Geometry check sheet. Reference: drawing and pictorial views, mm from the part's lowest x, y, z. A direction names the side the tool comes from. Coordinates: 2 decimals unless noted, no trailing zeros. Write each loop counter-clockwise with the first axis right and the second up, starting at its lowest first coordinate (ties: lowest second). Pieces come first, ordered by that corner, then holes. Notation, with made-up numbers: (58, 78) - (114, 78) arc R23 cw to (114, 99) - close; hole circle Ø2 at (4.5, 42). An arc over 180 degrees is marked (long way). Use one line per item in the form item = value. Start each with the question number.
(1) Sectioned sample at A-A (x = 7.5). Record the cut outline in (y, z).
(2) Gauge pin test, flat ends, axial feed: pin 1 Ø5.5 at (y, z) = (4, 7.5) entering from -X; pin 2 Ø6 at (x, y) = (7, 10.5) entering from +Z; pin 3 Ø8 at (x, z) = (4.5, 8.5) entering from -Y; pin 4 Ø6.5 at (y, z) = (4, 9) entering from -X. Record the tip position at first contact, or that the pin passes through.
(3) Material ranges on line 1 (Y direction, x = 15.1, z = 7.5); line 2 (X direction, y = 2.5, z = 6.5); line 3 (Y direction, x = 14, z = 9.5), recorded low to high. Write a range as [from, to].
(4) Tool access check on the marked faces 1 and 2. Record the directions out of +Z, -Z, +X, -X, +Y, -Y that give a thin tool (end or side, any length) a straight path to the whole face; none if there is none.
(5) Sectioned sample at B-B (y = 6.5). Record the cut outline in (x, z).
(6) Mould release check, pull along Z, two halves, no side actions. Record for the marked faces 3 and 4: released by +Z, released by -Z, zero draft, split by the parting line, or undercut.
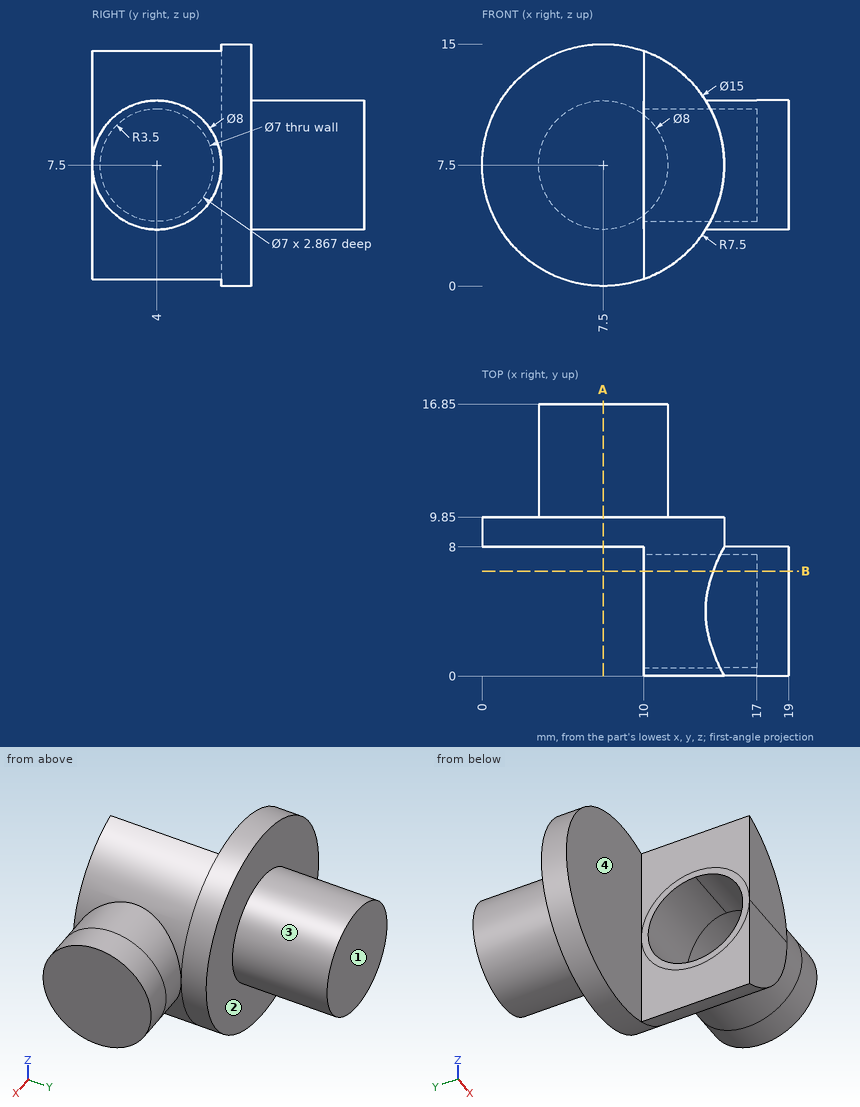
Answers below:
q1.outline = (8, 0) - (9.85, 0) - (9.85, 3.5) - (16.85, 3.5) - (16.85, 11.5) - (9.85, 11.5) - (9.85, 15) - (8, 15) - close
q2.pin_1 = 17
q2.pin_2 = 15
q2.pin_3 = 8
q2.pin_4 = 10
q3.line_1 = [0, 0.5], [7.5, 8]
q3.line_2 = [17, 19]
q3.line_3 = [0, 1.13], [6.87, 9.85]
q4.face_1 = +Z, -Z, +X, -X, +Y
q4.face_2 = +Y
q5.outline = (10, 0.43) arc R7.5 ccw to (14.32, 4.38) - (19, 4.38) - (19, 10.62) - (14.32, 10.62) arc R7.5 ccw to (10, 14.57) - (10, 9.95) - (17, 9.95) - (17, 5.05) - (10, 5.05) - close
q6.face_3 = split by the parting line
q6.face_4 = zero draft
